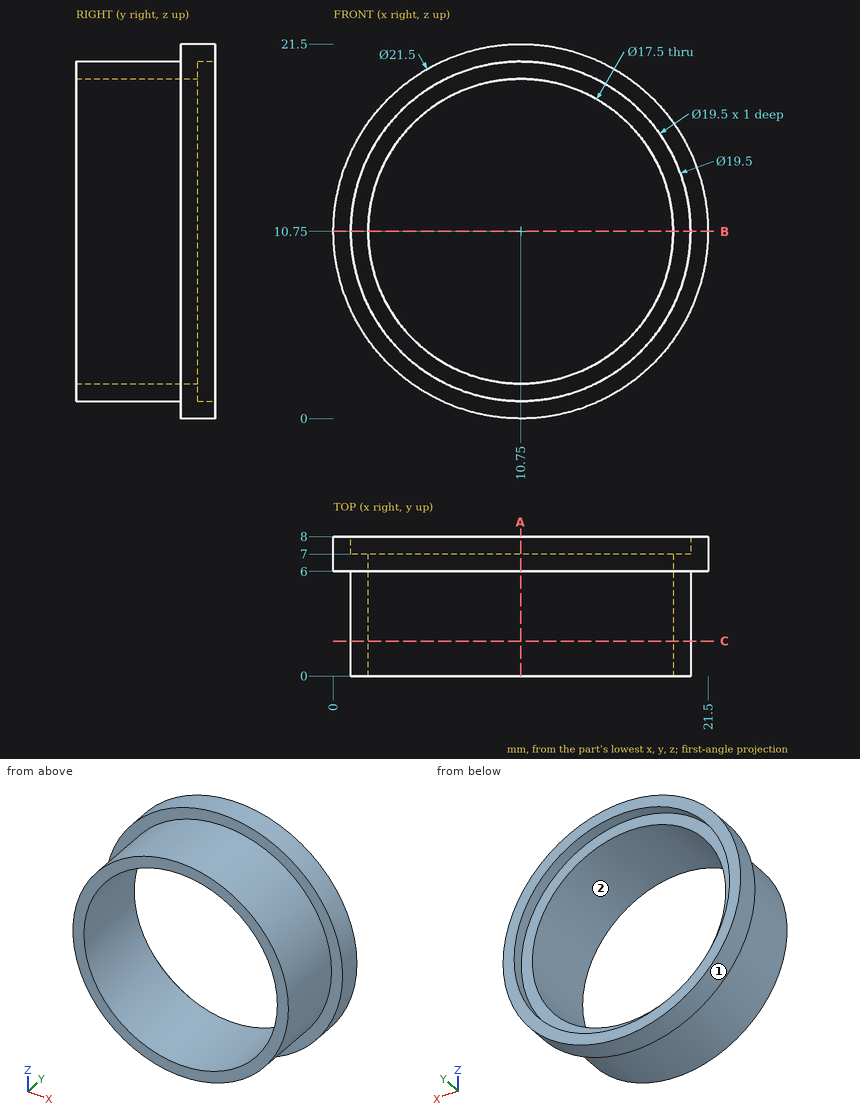
Part print with two shaded views. Sizes in mm from the minimum x, y, z corner. Round coordinates to 2 decimals unless told otherwise and drop trailing zeros. Order: outer loops, then holes, each group sorted by start corner. A loop starts at its lowest first (then second) coordinate and runs counter-clockwise, first axis right, second up. Notation, with made-up numbers: (57, 71) -> (107, 71) arc R19 ccw to (107, 106) -> close; hole circle Ø1 at (57, 41). An arc over 180 degrees is marked (long way). Write each question's results on one line, items separated by ' | '.
1. Wall check: line 1 along Z through (x, y) = (10.75, 7.2); line 2 along Y through (x, z) = (15.75, 2.75); line 3 along Z through (x, y) = (10.75, 2.5). Give the ranges that are in metal, low to high. Write a range as [from, to].
Findings below:
line 1: z = [0, 1], [20.5, 21.5] | line 2: y = [0, 7] | line 3: z = [1, 2], [19.5, 20.5]
2. Cut at B-B (z = 10.75). Give the cut face in (x, y).
Findings below:
outline: (0, 6) -> (1, 6) -> (1, 0) -> (2, 0) -> (2, 7) -> (1, 7) -> (1, 8) -> (0, 8) -> close; (19.5, 0) -> (20.5, 0) -> (20.5, 6) -> (21.5, 6) -> (21.5, 8) -> (20.5, 8) -> (20.5, 7) -> (19.5, 7) -> close
3. Flat gauge pins, fed straight in: P1, Ø3, axis at x = 8.5, y = 6.5, coming from the +Z side; P2, Ø1, axis at x = 4.5, y = 4, coming from the +Z side; P3, Ø10, axis at x = 12, z = 15, coming from the +Y side. Where does each tip first touch, or does it go through?
Findings below:
P1: stops at z = 21.47 | P2: stops at z = 18.62 | P3: stops at y = 7
4. Cut at C-C (y = 2). Give the cut face in (x, z), plus the area to 3 significant figures.
Findings below:
outline: circle Ø19.5 at (10.75, 10.75); hole circle Ø17.5 at (10.75, 10.75) | area: 58.1 mm²
5. Pull direction Z, two halves, no side cores. Call the marked faces 1 and 2: pulls with the +Z half, pulls with the -Z half, needs draft (parallel to the pull), parting line crosses it, or undercut.
Findings below:
face 1: parting line crosses it | face 2: undercut
6. Cut at A-A (x = 10.75). Give the cut face in (y, z).
Findings below:
outline: (0, 1) -> (6, 1) -> (6, 0) -> (8, 0) -> (8, 1) -> (7, 1) -> (7, 2) -> (0, 2) -> close; (0, 19.5) -> (7, 19.5) -> (7, 20.5) -> (8, 20.5) -> (8, 21.5) -> (6, 21.5) -> (6, 20.5) -> (0, 20.5) -> close
